Can you work these out from the model? Positions are in its coordinate system, mm. A direction names the side the tool comes from. Coordinates: 2 decimals unless noted, no trailing zeros. Order: outer loops, then holes, each group sorted by start corner. A loop starts at its lowest first (then second) coordinate and runs counter-clockwise, first axis right, second up.
Autodesk Inventor part; units mm, degrees
ref_plane "Work Plane1" through (2.1546, 0, 0.599) normal (1, 0, 0) x (0, 0, -1)
ref_plane "Work Plane2" through (0.8846, 0, 0.599) normal (1, 0, 0) x (0, 0, -1)
ref_plane "YZ Plane" through (0, 0, 0) normal (1, 0, 0) x (0, 1, 0)
sketch "Sketch1" plane through (0, 0, 0) normal (0, 1, 0) x (-1, 0, 0)
  line L0 (-2.7896, 0.599) -> (2.2904, 0.599)
  line L1 (2.2904, 0.599) -> (2.2904, -1.881)
  line L2 (2.2904, -1.881) -> (-2.7896, -1.881)
  line L3 (-2.7896, -1.881) -> (-2.7896, 0.599)
  point P0 (0, 0)
  dimension "d0" = 5.08
  dimension "d1" = 2.48
extrude "Extrusion1" add sketch "Sketch1" along normal blind 2.54
ref_plane "Work Plane1" through (2.1546, 0, 0.599) normal (1, 0, 0) x (0, 0, -1)
sketch "Sketch2" plane through (2.1546, 0, 0.599) normal (1, 0, 0) x (0, 0, -1)
  line L0 (0.99, 8.38) -> (1.47, 8.38)
  line L1 (1.47, 8.38) -> (1.47, -0.79)
  line L2 (0.99, -0.142) -> (0.99, 8.38)
  line L3 (3.75, -0.79) -> (1.47, -0.79)
  line L4 (0.99, -0.142) -> (0.99, -1.27)
  line L5 (0.99, -1.27) -> (3.75, -1.27)
  line L6 (3.75, -1.27) -> (3.75, -0.79)
  line L7 (0, 2.54) -> (2.48, 2.54)
  line L8 (2.48, 0) -> (0, 0)
  line L9 (2.48, 0) -> (2.48, 2.54)
  point P0 (0.599, 0)
  dimension "d5" = 0.48
  dimension "d6" = 0.48
  dimension "d7" = 5.84
  dimension "d8" = 1.27
  dimension "d9" = 1.01
  dimension "d10" = 1.27
extrude "Extrusion2" add sketch "Sketch2" along normal mid plane 0.46 contours L0 L1 L7 L2 | L7 L1 L8 L2 | L8 L1 L3 L6 L5 L4 L2
pattern_linear "Rectangular Pattern1" count 2 spacing 2.54 along (-1, 0, 0) of "Extrusion2"
ref_plane "Work Plane2" through (0.8846, 0, 0.599) normal (1, 0, 0) x (0, 0, -1)
sketch "Sketch3" plane through (0.8846, 0, 0.599) normal (1, 0, 0) x (0, 0, -1)
  line L0 (0.99, 8.38) -> (1.47, 8.38)
  line L1 (1.47, 8.38) -> (1.47, -0.79)
  line L2 (0.99, -0.142) -> (0.99, 8.38)
  line L3 (0.99, -0.142) -> (0.99, -0.79)
  line L4 (1.47, 8.38) -> (0.99, 8.38)
  line L5 (0.99, 8.38) -> (0.99, -0.79)
  line L6 (1.47, -0.142) -> (1.47, 8.38)
  line L7 (-1.29, -0.79) -> (0.99, -0.79)
  line L8 (1.47, -0.142) -> (1.47, -1.27)
  line L9 (1.47, -1.27) -> (-1.29, -1.27)
  line L10 (-1.29, -1.27) -> (-1.29, -0.79)
  point P0 (0.599, 0)
  dimension "d18" = 0.48
extrude "Extrusion3" add sketch "Sketch3" along normal mid plane 0.46
pattern_linear "Rectangular Pattern2" count 2 spacing 2.54 along (-1, 0, 0) of "Extrusion3"
properties part number "Header_127"
1. Imagine slicing it at D-D on x = -0.4. Please give me the cut outline in (y, z).
Completed:
outline: (-1.27, -3.15) - (-0.79, -3.15) - (-0.79, -0.87) - (0, -0.87) - (0, -1.88) - (2.54, -1.88) - (2.54, -0.87) - (8.38, -0.87) - (8.38, -0.39) - (2.54, -0.39) - (2.54, 0.6) - (0, 0.6) - (0, -0.39) - (-1.27, -0.39) - close
2. On a 3-axis mill with a long thin cutter (end or side, diameter ignored), from which of +Z, -Z, +X, -X, +Y, -Y can I reach the whole of each face in a straight line? I mean faces 3 (the flat face through (-0.155, -1, -1)), 4 (the flat face through (-1.885, -1, 0)), 5 (the flat face through (2.79, 1, -1)), 6 (the flat face through (-2.29, 1, -1)), 7 (the flat face through (2.385, -1, -1)). Say none if no direction works.
Completed:
face 3: +Z, -Z, -Y
face 4: +Z, -Z, -X, -Y
face 5: +Z, -Z, +X, +Y, -Y
face 6: +Z, -Z, -X, +Y, -Y
face 7: +Z, -Z, +X, -Y
3. Please list where these lines run through material, in increasing order: probe 1 along X at (y, z) = (7.25, -0.8); probe 2 along Y at (x, z) = (0.1, 0); probe 3 along Z at (x, y) = (-0.75, 2.5).
Completed:
probe 1: x = -1.89 to -1.43, -0.62 to -0.16, 0.65 to 1.11, 1.92 to 2.38
probe 2: y = 0 to 2.54
probe 3: z = -1.88 to 0.6
4. Imagine slicing it at C-C on z = -1. Please give me the cut outline in (x, y).
Completed:
outline: (-2.29, 0) - (2.79, 0) - (2.79, 2.54) - (-2.29, 2.54) - close; (-0.62, -1.27) - (-0.16, -1.27) - (-0.16, -0.79) - (-0.62, -0.79) - close; (1.92, -1.27) - (2.38, -1.27) - (2.38, -0.79) - (1.92, -0.79) - close
5. I'm going to push flat-ended pins straight in: pin 1 (1 mm diameter, centred on x = -0.5, z = -1.5, fed in from +Y); pin 2 (1.4 mm diameter, centred on y = -1, z = -1.5, fed in from +X); pin 3 (2 mm diameter, centred on x = 0, y = 1.5, fed in from +Z). Where does each tip first touch, or does it pass through?
Completed:
pin 1: stops at y = 2.54
pin 2: stops at x = 2.38
pin 3: stops at z = 0.6
6. Imagine slicing it at B-B on z = 1.3. Please give me the cut outline in (x, y).
Completed:
outline: (-1.89, -1.27) - (-1.43, -1.27) - (-1.43, -0.79) - (-1.89, -0.79) - close; (0.65, -1.27) - (1.11, -1.27) - (1.11, -0.79) - (0.65, -0.79) - close
7. Thinking about a two-plate mould opening in Y: for faces 1 (the flat face through (0, 0, -1)), 2 (the flat face through (0, 1, 0.599)), which applies, pulls with the +Y half, pulls with the -Y half, needs draft (parallel to the pull), parting line crosses it, or undercut?
Completed:
face 1: undercut
face 2: needs draft
8. Imagine slicing it at A-A on y = -0.25. Please give me the cut outline in (x, z).
Completed:
outline: (-1.89, -0.87) - (-1.43, -0.87) - (-1.43, -0.39) - (-1.89, -0.39) - close; (-0.62, -0.87) - (-0.16, -0.87) - (-0.16, -0.39) - (-0.62, -0.39) - close; (0.65, -0.87) - (1.11, -0.87) - (1.11, -0.39) - (0.65, -0.39) - close; (1.92, -0.87) - (2.38, -0.87) - (2.38, -0.39) - (1.92, -0.39) - close
